Part model, mm, in its own coordinate system. Face numbers are marked on the shaded views. Coordinates: 2 decimals unless noted, no trailing zeros. Write each loop counter-clockwise with the first axis right and the second up, starting at its lowest first coordinate (ties: lowest second). Pieces come first, ordered by that corner, then holes. Notation, with made-up numbers: (-9.75, 63) -> (36.25, 63) arc R27 ccw to (36.25, 88) -> close; hole circle Ø3 at (64.5, 73.5). An arc over 180 degrees is marked (long way). Write item = value, one per line. Start each with the question number.
Q1. Band-saw the part on D-D, the plane z = 14.4. List the corners of the cut face in (x, y), plus the area to 3 significant figures.
Q2. Pull direction X, two halves, no side cores. Call the marked faces 1, 2 and 3: released by +X, released by -X, zero draft, split by the parting line, or undercut.
Q3. Pin check, flat tips, straight feed: P1, Ø8, axis at x = -6.5, y = 10, coming from the +Z side; P2, Ø8, axis at y = 15, z = -1.5, coming from the -X side; P3, Ø1, axis at x = -21.5, y = 3, coming from the +Z side. Stop position of each tip, or through.
Q4. Probe line 1 (X direction, y = 1.7, z = 14.4); line 2 (Y direction, x = 11, z = 12); line 3 (Z direction, x = -25, y = 1). List the from-to ranges inside material, lowest first.
Q5. Band-saw the part on C-C, the plane y = 2.75. List the corners of the cut face in (x, z).
Q6. Band-saw the part on B-B, the plane x = 0. Give the number of separate pieces and of enclosed holes in the cut face, plus the area to 3 significant figures.
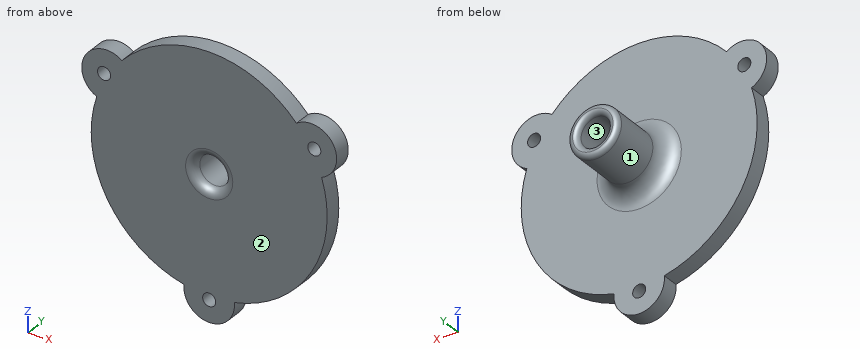
from build123d import *

# Parameters (mm, degrees)
SKETCH1_R           = 28
BOSS_EXTRUDE1_DEPTH = 4
SKETCH2_R           = 6
BOSS_EXTRUDE2_DEPTH = 4
SKETCH3_R           = 1.55
CUT_EXTRUDE1_DEPTH  = 46.683525867
SKETCH4_R           = 3.6
CUT_EXTRUDE2_DEPTH  = 46.683525867
BOSS_EXTRUDE3_START = 16
SKETCH5_R           = 6
SKETCH5_R_2         = 3.6
BOSS_EXTRUDE3_DEPTH = 16
FILLET1_R           = 4
FILLET2_R           = 1.2
FILLET3_R           = 2


with BuildPart() as part:
    # Sketch1 → Boss-Extrude1 (new body)
    with BuildSketch(Plane(origin=(0, 0, 0), x_dir=(1, 0, 0), z_dir=(0, 1, 0))):
        with Locations(Location((0, 0, 0), (0, 0, 270))):
            Circle(SKETCH1_R)
    extrude(amount=BOSS_EXTRUDE1_DEPTH)

    # Sketch2 → Boss-Extrude2 (add)
    with BuildSketch(Plane(origin=(0, 4, 0), x_dir=(1, 0, 0), z_dir=(0, 1, 0))):
        with Locations((0, 28)):
            Circle(SKETCH2_R)
        with Locations((24.248711306, -14)):
            Circle(SKETCH2_R)
        with Locations((-24.248711306, -14)):
            Circle(SKETCH2_R)
    extrude(amount=-BOSS_EXTRUDE2_DEPTH)

    # Sketch3 → Cut-Extrude1 (cut, through all)
    with BuildSketch(Plane(origin=(0, 4, 0), x_dir=(1, 0, 0), z_dir=(0, 1, 0))):
        with Locations(Location((0, 28.8, 0), (0, 0, 270))):
            Circle(SKETCH3_R)
        with Locations(Location((24.941531629, -14.4, 0), (0, 0, 270))):
            Circle(SKETCH3_R)
        with Locations(Location((-24.941531629, -14.4, 0), (0, 0, 270))):
            Circle(SKETCH3_R)
    extrude(amount=-CUT_EXTRUDE1_DEPTH, mode=Mode.SUBTRACT)

    # Sketch4 → Cut-Extrude2 (cut, through all)
    with BuildSketch(Plane(origin=(0, 4, 0), x_dir=(1, 0, 0), z_dir=(0, 1, 0))):
        with Locations(Location((0, 0, 0), (0, 0, 270))):
            Circle(SKETCH4_R)
    extrude(amount=-CUT_EXTRUDE2_DEPTH, mode=Mode.SUBTRACT)

    # Sketch5 → Boss-Extrude3 (add)
    with BuildSketch(Plane(origin=(0, 4, 0), x_dir=(1, 0, 0), z_dir=(0, 1, 0)).offset(BOSS_EXTRUDE3_START)):
        with Locations(Location((0, 0, 0), (0, 0, 270))):
            Circle(SKETCH5_R)
        with Locations(Location((0, 0, 0), (0, 0, 270))):
            Circle(SKETCH5_R_2, mode=Mode.SUBTRACT)
    extrude(amount=-BOSS_EXTRUDE3_DEPTH)

    # Fillet1
    fillet1_edges = [part.edges().sort_by_distance(p)[0] for p in [
        (0, 4, -6),
    ]]
    fillet(fillet1_edges, radius=FILLET1_R)

    # Fillet2
    fillet2_edges = [part.edges().sort_by_distance(p)[0] for p in [
        (0, 20, -6),
        (0, 20, -3.6),
    ]]
    fillet(fillet2_edges, radius=FILLET2_R - 0.0001)  # a hair under: the kernel refuses the full size

    # Fillet3
    fillet3_edges = [part.edges().sort_by_distance(p)[0] for p in [
        (0, 0, -3.6),
    ]]
    fillet(fillet3_edges, radius=FILLET3_R)


solid = part.part
Ans:
q1.outline = (-30.24, 0) -> (-26.49, 0) -> (-26.49, 4) -> (-30.24, 4) -> close; (-23.39, 0) -> (23.39, 0) -> (23.39, 4) -> (-23.39, 4) -> close; (26.49, 0) -> (30.24, 0) -> (30.24, 4) -> (26.49, 4) -> close
q1.area = 217 mm2
q2.face_1 = split by the parting line
q2.face_2 = zero draft
q2.face_3 = undercut
q3.P1 = 5.45
q3.P2 = -6
q3.P3 = 19.56
q4.line_1 = -30.24 to -26.49, -23.39 to 23.39, 26.49 to 30.24
q4.line_2 = 0 to 4
q4.line_3 = -12.61 to 12.85, 15.95 to 19.95
q5.outline = (-26.67, 8.51) arc R28 ccw to (-5.97, -27.36) arc R6 ccw (long way) to (5.97, -27.36) arc R28 ccw to (26.67, 8.51) arc R6 ccw (long way) to (20.71, 18.84) arc R28 ccw to (-20.71, 18.84) arc R6 ccw (long way) to start; hole circle Ø3.1 at (-24.94, 14.4); hole circle Ø7.2 at (0, 0); hole circle Ø3.1 at (0, -28.8); hole circle Ø3.1 at (24.94, 14.4)
q6.separate_pieces = 3
q6.enclosed_holes = 0
q6.area = 288 mm2
